Build history of the part. All positions in model axes, mm. Face numbers are marked on the shaded views. A direction names the side the tool comes from. Round coordinates to 2 decimals unless told otherwise and drop trailing zeros. Write each loop counter-clockwise with the first axis right and the second up, starting at its lowest first coordinate (ties: lowest second). Pieces come first, ordered by that corner, then holes. Notation, with made-up numbers: (63.25, 76.25) -> (104.25, 76.25) arc R24 ccw to (104.25, 113.25) -> close; hole circle Ø1 at (55.5, 42). An arc over 180 degrees is marked (long way). Answer as CSV lines item,"result".
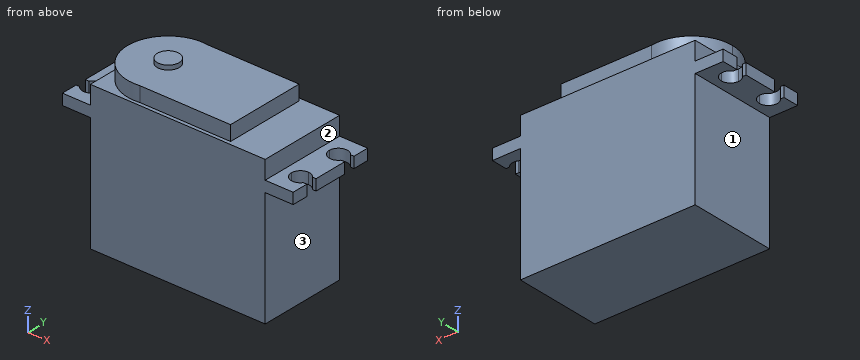
from build123d import *

# Parameters (mm, degrees)
F0_W      = 40
F0_H      = 20
F1_DEPTH  = 26.5
F2_W      = 52.8
F2_H      = 20
F3_DEPTH  = 2.5
F4_W      = 40
F4_H      = 20
F5_DEPTH  = 4.2
F7_DEPTH  = 3.4
F8_R      = 2.5
F9_DEPTH  = 1
F11_DEPTH = 29.001


with BuildPart() as f1:
    # F0 (on Top) → F1 (new body)
    with BuildSketch(Plane.XY):
        Rectangle(F0_W, F0_H)
    extrude(amount=F1_DEPTH)

    # F2 (on face) → F3 (join)
    with BuildSketch(Plane.XY.offset(26.5)):
        Rectangle(F2_W, F2_H)
    extrude(amount=F3_DEPTH)

    # F4 (on face) → F5 (join)
    with BuildSketch(Plane.XY.offset(29)):
        Rectangle(F4_W, F4_H)
    extrude(amount=F5_DEPTH)

    # F6 (on face) → F7 (join)
    with BuildSketch(Plane.XY.offset(33.2)):
        with BuildLine():
            Line((-10.7, 9.2), (-9.3398529491, 9.2))
            ThreePointArc((-9.3398529491, 9.2), (-16.7762090282, 7.0405741134), (-20, 1.29e-08))
            ThreePointArc((-20, 1.29e-08), (-16.7762090379, -7.040574105), (-9.3398529491, -9.2))
            Line((-9.3398529491, -9.2), (-10.7, -9.2))
            Line((-10.7, -9.2), (-10.7, 9.2))
        make_face()
        with BuildLine():
            ThreePointArc((-9.3398529491, -9.2), (-3.6594258908, -6.0762090331), (-1.4, 0))
            ThreePointArc((-1.4, 0), (-3.6594258908, 6.0762090331), (-9.3398529491, 9.2))
            Line((-9.3398529491, 9.2), (-10.7, 9.2))
            Line((-10.7, 9.2), (-10.7, -9.2))
            Line((-10.7, -9.2), (-9.3398529491, -9.2))
        make_face()
        with BuildLine():
            ThreePointArc((-9.3398529491, 9.2), (-3.6594258908, 6.0762090331), (-1.4, 0))
            ThreePointArc((-1.4, 0), (-3.6594258908, -6.0762090331), (-9.3398529491, -9.2))
            Line((-9.3398529491, -9.2), (11.4008062363, -9.2))
            Line((11.4008062363, -9.2), (11.4008062363, 9.2))
            Line((11.4008062363, 9.2), (-9.3398529491, 9.2))
        make_face()
    extrude(amount=F7_DEPTH)

    # F8 (on face) → F9 (join)
    with BuildSketch(Plane.XY.offset(36.6)):
        with Locations((-10.7, 0)):
            Circle(F8_R)
    extrude(amount=F9_DEPTH)

    # F10 (on face) → F11 (cut, through all)
    with BuildSketch(Plane.XY.offset(29)):
        with BuildLine():
            Line((-23.9, 3), (-23.9, 5.1))
            Line((-23.9, 5.1), (-21.8, 5.1))
            ThreePointArc((-21.8, 5.1), (-23.2478597857, 7.0961746268), (-25.594964896, 6.3397959514))
            Line((-25.594964896, 6.3397959514), (-24.7499752088, 6.3397959514))
            Line((-24.7499752088, 6.3397959514), (-24.7499752088, 3.8397959514))
            Line((-24.7499752088, 3.8397959514), (-25.5798469442, 3.8397959514))
            ThreePointArc((-25.5798469442, 3.8397959514), (-24.839034477, 3.2216458665), (-23.9, 3))
        make_face()
        with BuildLine():
            Line((-21.8, 5.1), (-23.9, 5.1))
            Line((-23.9, 5.1), (-23.9, 3))
            ThreePointArc((-23.9, 3), (-22.4150757595, 3.6150757595), (-21.8, 5.1))
        make_face()
        with BuildLine():
            Line((-24.7499752088, 6.3397959514), (-25.594964896, 6.3397959514))
            ThreePointArc((-25.594964896, 6.3397959514), (-25.9999616042, 5.0873011527), (-25.5798469442, 3.8397959514))
            Line((-25.5798469442, 3.8397959514), (-24.7499752088, 3.8397959514))
            Line((-24.7499752088, 3.8397959514), (-24.7499752088, 6.3397959514))
        make_face()
        with BuildLine():
            Line((-23.9, -5.1), (-23.9, -3))
            ThreePointArc((-23.9, -3), (-24.839034477, -3.2216458665), (-25.5798469442, -3.8397959514))
            Line((-25.5798469442, -3.8397959514), (-24.7499752088, -3.8397959514))
            Line((-24.7499752088, -3.8397959514), (-24.7499752088, -6.3397959514))
            Line((-24.7499752088, -6.3397959514), (-25.594964896, -6.3397959514))
            ThreePointArc((-25.594964896, -6.3397959514), (-23.2478597857, -7.0961746268), (-21.8, -5.1))
            Line((-21.8, -5.1), (-23.9, -5.1))
        make_face()
        with BuildLine():
            ThreePointArc((-21.8, -5.1), (-22.4150757595, -3.6150757595), (-23.9, -3))
            Line((-23.9, -3), (-23.9, -5.1))
            Line((-23.9, -5.1), (-21.8, -5.1))
        make_face()
        with BuildLine():
            Line((-24.7499752088, -3.8397959514), (-25.5798469442, -3.8397959514))
            ThreePointArc((-25.5798469442, -3.8397959514), (-25.9999616042, -5.0873011527), (-25.594964896, -6.3397959514))
            Line((-25.594964896, -6.3397959514), (-24.7499752088, -6.3397959514))
            Line((-24.7499752088, -6.3397959514), (-24.7499752088, -3.8397959514))
        make_face()
        with BuildLine():
            ThreePointArc((26, 5.1), (25.8961746268, 5.7521402143), (25.594964896, 6.3397959514))
            Line((25.594964896, 6.3397959514), (24.7499752088, 6.3397959514))
            Line((24.7499752088, 6.3397959514), (24.7499752088, 3.8397959514))
            Line((24.7499752088, 3.8397959514), (25.5798469442, 3.8397959514))
            ThreePointArc((25.5798469442, 3.8397959514), (25.8921945918, 4.4358007012), (26, 5.1))
        make_face()
        with BuildLine():
            ThreePointArc((25.594964896, 6.3397959514), (23.2478597857, 7.0961746268), (21.8, 5.1))
            Line((21.8, 5.1), (23.9, 5.1))
            Line((23.9, 5.1), (23.9, 3))
            ThreePointArc((23.9, 3), (24.839034477, 3.2216458665), (25.5798469442, 3.8397959514))
            Line((25.5798469442, 3.8397959514), (24.7499752088, 3.8397959514))
            Line((24.7499752088, 3.8397959514), (24.7499752088, 6.3397959514))
            Line((24.7499752088, 6.3397959514), (25.594964896, 6.3397959514))
        make_face()
        with BuildLine():
            Line((23.9, 5.1), (21.8, 5.1))
            ThreePointArc((21.8, 5.1), (22.4150757595, 3.6150757595), (23.9, 3))
            Line((23.9, 3), (23.9, 5.1))
        make_face()
        with BuildLine():
            Line((27.2499752088, 6.3397959514), (25.594964896, 6.3397959514))
            ThreePointArc((25.594964896, 6.3397959514), (25.8961746268, 5.7521402143), (26, 5.1))
            ThreePointArc((26, 5.1), (25.8921945918, 4.4358007012), (25.5798469442, 3.8397959514))
            Line((25.5798469442, 3.8397959514), (27.2499752088, 3.8397959514))
            Line((27.2499752088, 3.8397959514), (27.2499752088, 6.3397959514))
        make_face()
        with BuildLine():
            ThreePointArc((26, -5.1), (25.8961746268, -5.7521402143), (25.594964896, -6.3397959514))
            Line((25.594964896, -6.3397959514), (27.2499752088, -6.3397959514))
            Line((27.2499752088, -6.3397959514), (27.2499752088, -3.8397959514))
            Line((27.2499752088, -3.8397959514), (25.5798469442, -3.8397959514))
            ThreePointArc((25.5798469442, -3.8397959514), (25.8921945918, -4.4358007012), (26, -5.1))
        make_face()
        with BuildLine():
            Line((23.9, -5.1), (21.8, -5.1))
            ThreePointArc((21.8, -5.1), (23.2478597857, -7.0961746268), (25.594964896, -6.3397959514))
            Line((25.594964896, -6.3397959514), (24.7499752088, -6.3397959514))
            Line((24.7499752088, -6.3397959514), (24.7499752088, -3.8397959514))
            Line((24.7499752088, -3.8397959514), (25.5798469442, -3.8397959514))
            ThreePointArc((25.5798469442, -3.8397959514), (24.839034477, -3.2216458665), (23.9, -3))
            Line((23.9, -3), (23.9, -5.1))
        make_face()
        with BuildLine():
            ThreePointArc((23.9, -3), (22.4150757595, -3.6150757595), (21.8, -5.1))
            Line((21.8, -5.1), (23.9, -5.1))
            Line((23.9, -5.1), (23.9, -3))
        make_face()
        with BuildLine():
            Line((24.7499752088, -6.3397959514), (25.594964896, -6.3397959514))
            ThreePointArc((25.594964896, -6.3397959514), (25.8961746268, -5.7521402143), (26, -5.1))
            ThreePointArc((26, -5.1), (25.8921945918, -4.4358007012), (25.5798469442, -3.8397959514))
            Line((25.5798469442, -3.8397959514), (24.7499752088, -3.8397959514))
            Line((24.7499752088, -3.8397959514), (24.7499752088, -6.3397959514))
        make_face()
        with BuildLine():
            ThreePointArc((-25.594964896, -6.3397959514), (-25.9999616042, -5.0873011527), (-25.5798469442, -3.8397959514))
            Line((-25.5798469442, -3.8397959514), (-26.4, -3.8397959514))
            Line((-26.4, -3.8397959514), (-26.4, -6.3397959514))
            Line((-26.4, -6.3397959514), (-25.594964896, -6.3397959514))
        make_face()
        with BuildLine():
            ThreePointArc((-25.5798469442, 3.8397959514), (-25.9999616042, 5.0873011527), (-25.594964896, 6.3397959514))
            Line((-25.594964896, 6.3397959514), (-26.4, 6.3397959514))
            Line((-26.4, 6.3397959514), (-26.4, 3.8397959514))
            Line((-26.4, 3.8397959514), (-25.5798469442, 3.8397959514))
        make_face()
    extrude(amount=-F11_DEPTH, mode=Mode.SUBTRACT)


solid = f1.part
1. Probe line 1 along X through (y, z) = (-0.25, 5.5); line 2 along Z through (x, y) = (8.5, 2.5); line 3 along Z through (x, y) = (14, -8.5). List the from-to ranges inside material, lowest first.
Results found:
line 1,"x = -20 to 20"
line 2,"z = 0 to 36.6"
line 3,"z = 0 to 33.2"
2. Cut at D-D, the plane x = 23. Write the cut outline in (y, z), then the cut area to 3 significant figures.
Results found:
outline,"(-10, 26.5) -> (-7, 26.5) -> (-7, 29) -> (-10, 29) -> close; (-3.2, 26.5) -> (3.2, 26.5) -> (3.2, 29) -> (-3.2, 29) -> close; (7, 26.5) -> (10, 26.5) -> (10, 29) -> (7, 29) -> close"
area,"31.0 mm2"
3. Cut at C-C, the plane y = 1.25. Write the cut outline in (x, z).
Results found:
outline,"(-26.4, 26.5) -> (-20, 26.5) -> (-20, 0) -> (20, 0) -> (20, 26.5) -> (26.4, 26.5) -> (26.4, 29) -> (20, 29) -> (20, 33.2) -> (11.4, 33.2) -> (11.4, 36.6) -> (-8.53, 36.6) -> (-8.53, 37.6) -> (-12.87, 37.6) -> (-12.87, 36.6) -> (-19.92, 36.6) -> (-19.92, 33.2) -> (-20, 33.2) -> (-20, 29) -> (-26.4, 29) -> close"
4. Which spindle directions (+Z, -Z, +X, -X, +Y, -Y) get a long thin tool onto all of the face, cutting with end or side? Do the marked faces 1, 2 and 3. Say none if no direction does.
Results found:
face 1,"-Z, -X, +Y, -Y"
face 2,"+Z, +X, +Y, -Y"
face 3,"-Z, +X, +Y, -Y"
5. Drop flat-ended pins along their axis: pin 1 Ø3.5 at (y, z) = (0, 31.5) entering from +X; pin 2 Ø2.5 at (x, z) = (2, 35) entering from +Y; pin 3 Ø7 at (x, y) = (22.5, 3) entering from +Z. Give the stop position or say it passes through.
Results found:
pin 1,"stops at x = 20"
pin 2,"stops at y = 9.2"
pin 3,"stops at z = 33.2"
6. Cut at B-B, the plane x = -6. Write the cut outline in (y, z).
Results found:
outline,"(-10, 0) -> (10, 0) -> (10, 33.2) -> (9.2, 33.2) -> (9.2, 36.6) -> (-9.2, 36.6) -> (-9.2, 33.2) -> (-10, 33.2) -> close"
7. Cut at A-A, the plane z = 28. Write the cut outline in (x, y).
Results found:
outline,"(-26.4, -10) -> (26.4, -10) -> (26.4, -6.34) -> (25.59, -6.34) arc R2.1 cw (long way) to (25.58, -3.84) -> (26.4, -3.84) -> (26.4, 3.84) -> (25.58, 3.84) arc R2.1 cw (long way) to (25.59, 6.34) -> (26.4, 6.34) -> (26.4, 10) -> (-26.4, 10) -> (-26.4, 6.34) -> (-25.59, 6.34) arc R2.1 cw (long way) to (-25.58, 3.84) -> (-26.4, 3.84) -> (-26.4, -3.84) -> (-25.58, -3.84) arc R2.1 cw (long way) to (-25.59, -6.34) -> (-26.4, -6.34) -> close"
